Autodesk Inventor part; units mm, degrees
ref_plane "YZ Plane" through (0, 0, 0) normal (1, 0, 0) x (0, 1, 0)
ref_plane "XZ Plane" through (0, 0, 0) normal (0, 1, 0) x (-1, 0, 0)
ref_plane "XY Plane" through (0, 0, 0) normal (0, 0, 1) x (1, 0, 0)
sketch "Szkic1" plane through (0, 0, 0) normal (0, 1, 0) x (-1, 0, 0)
  line L0 (30.1, 0) -> (-30.1, 0)
  circle A0 centre (0, 0) radius 18
  circle A1 centre (0, 0) radius 21.5
  line L1 (17.9892, -0.6225) -> (21.3298, -2.7)
  line L2 (17.9892, 0.6225) -> (21.3298, 2.7)
  point P0 (21.3298, 2.7)
  point P1 (17.9892, 0.6225)
  dimension "d4" = 43
  dimension "d5" = 36
  dimension "d6" = 5.4
  dimension "d7" = 1.245
sketch3d "Szkic 3D2"
  line L0 (18, 15, 0) -> (18, -15, 0)
  arc A0 (18, -15, 0) -> (8, -25, 0) centre (8, -15, 0) ccw
  line L1 (8, -25, 0) -> (-8, -25, 0)
  arc A1 (-8, -25, 0) -> (-18, -15, 0) centre (-8, -15, 0) ccw
  line L2 (-18, -15, 0) -> (-18, 15, 0)
  arc A2 (-18, 15, 0) -> (-8, 25, 0) centre (-8, 15, 0) ccw
  line L3 (-8, 25, 0) -> (8, 25, 0)
  arc A3 (8, 25, 0) -> (18, 15, 0) centre (8, 15, 0) ccw
  dimension "d9" = 50
  dimension "d10" = 36
  dimension "d11" = 10
  dimension "d12" = 10
  dimension "d13" = 10
  dimension "d14" = 10
sweep "Przeciągnięcie2" add profiles "Szkic1" path "Szkic 3D2" picked at (20.2478, -1.7084) picked at (20.2478, 1.7084) contours A1 L1 A0 L0 | L0 A0 L2 A1
equation "\"d12\" = d11"
equation "\"d13\" = d11"
equation "\"d14\" = d11"
properties part number "single_coil"
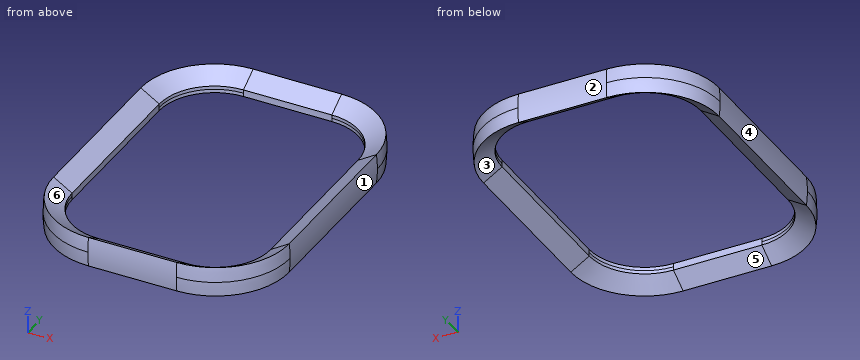
Geometry: final body of the model. Coordinates: model frame, mm. Face numbers are marked on the shaded views. A direction names the side the tool comes from. Give positions to 0.01 mm unless a question says otherwise; leave off trailing zeros. Loops run counter-clockwise (first coordinate to the right, second up) from the corner with the lowest first, then second, coordinate; pieces in that order, holes last. Notation, with made-up numbers: (-18.5, 53.25) - (1.5, 53.25) arc R19 ccw to (1.5, 60.25) - close; hole circle Ø8 at (45, -37). An arc over 180 degrees is marked (long way). Answer as CSV lines item,"result". Start each with the question number.
1. Pin query (flat end, axial travel): P1, Ø3, axis at x = 16.5, z = 1.5, coming from the +Y side; P2, Ø2, axis at x = -7, z = -1.5, coming from the -Y side; P3, Ø3, axis at x = 13, z = 1.5, coming from the +Y side. Return the tip coordinate at first contact, or that it passes through.
2. Ray query, L1, parallel to X at y = 15, z = 0.25; L2, parallel to Y at x = -7, z = 0.5; L3, parallel to Y at x = 17, z = 2. Return the intervals inside material, ascending.
3. Reachability of the marked faces 4, 5 and 6 from +Z, -Z, +X, -X, +Y, -Y: full face, straight path, thin tool, end or side. Return the list, or none.
4. Section B-B, the plane x = -0.5. Return loops of the section in (y, z).
5. Section A-A, the plane y = -4. Return loops of the section in (x, z), plus the area to 3 significant figures.
6. Draft query along X for the marked faces 1, 2 and 3. Return one class per face: released by +X, released by -X, zero draft, split by the parting line, or undercut.
Answers:
1,P1,"stops at y = 26.49"
1,P2,"stops at y = -28.49"
1,P3,"stops at y = 28"
2,L1,"x = -21.5 to -18, 18 to 21.5"
2,L2,"y = -28.49 to -24.99, 24.99 to 28.49"
2,L3,"y = -24.94 to -23.24, 23.24 to 24.94"
3,face 4,"-X, +Y, -Y"
3,face 5,"-Z"
3,face 6,"+Z"
4,outline,"(-28.33, -2.7) - (-24.99, -0.62) arc R18 cw to (-24.99, 0.62) - (-28.33, 2.7) arc R21.5 ccw to start; (24.99, -0.62) - (28.33, -2.7) arc R21.5 ccw to (28.33, 2.7) - (24.99, 0.62) arc R18 cw to start"
5,outline,"(-21.33, -2.7) - (-17.99, -0.62) arc R18 cw to (-17.99, 0.62) - (-21.33, 2.7) arc R21.5 ccw to start; (17.99, -0.62) - (21.33, -2.7) arc R21.5 ccw to (21.33, 2.7) - (17.99, 0.62) arc R18 cw to start"
5,area,"23.4 mm2"
6,face 1,"released by +X"
6,face 2,"zero draft"
6,face 3,"undercut"
